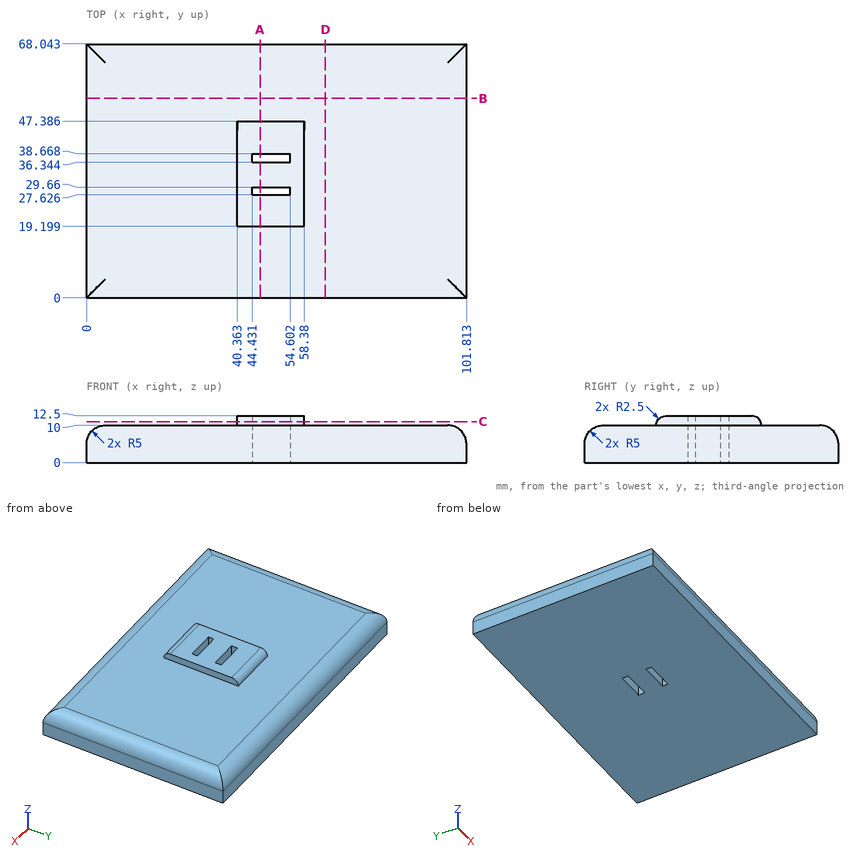
Geometry: see drawing. Coordinates: mm, zero at the bounding-box minimum. Coordinates: 2 decimals unless noted, no trailing zeros. Loops run counter-clockwise (first coordinate to the right, second up) from the corner with the lowest first, then second, coordinate; pieces in that order, holes last. Notation, with made-up numbers: (-11.75, -6) - (43.25, -6) arc R20 cw to (43.25, 1) - close; hole circle Ø4 at (-14.75, 73). An arc over 180 degrees is marked (long way). Put each result on its own line as item: value. Start each with the question number.
Q1. Cut plane C-C, the plane z = 11. Return loops of the section in (x, y).
Q2. Line query: line 1 (Y direction, x = 51.5, z = 2.5); line 2 (X direction, y = 28.5, z = 1); line 3 (X direction, y = 22, z = 11). Output: solid intervals per line, ascending.
Q3. Cut plane A-A, the plane x = 46.5. Give the number of separate pieces and of enclosed holes in the cut face, and give its area (3 significant figures).
Q4. Cut plane D-D, the plane x = 64. Return loops of the section in (y, z).
Q5. Cut plane B-B, the plane y = 53.5. Return loops of the section in (x, z), and give its area (3 significant figures).
Q6. Pin query (flat end, axial travel): pin 1 Ø3 at (x, z) = (31.5, 8) entering from +Y; pin 2 Ø5 at (x, y) = (27.5, 24) entering from +Z; pin 3 Ø1.2 at (y, z) = (38, 9) entering from +X. Return the tip coordinate at first contact, or that it passes through.
Filled sheet:
1. outline: (40.36, 19.41) - (58.38, 19.41) - (58.38, 47.18) - (40.36, 47.18) - close; hole (44.43, 27.63) - (54.6, 27.63) - (54.6, 29.66) - (44.43, 29.66) - close; hole (44.43, 36.34) - (54.6, 36.34) - (54.6, 38.67) - (44.43, 38.67) - close
2. line 1: 0 to 27.63, 29.66 to 36.34, 38.67 to 68.04
2. line 2: 0 to 44.43, 54.6 to 101.81
2. line 3: 40.36 to 58.38
3. separate pieces: 3
3. enclosed holes: 0
3. area: 683 mm²
4. outline: (0, 0) - (68.04, 0) - (68.04, 5) arc R5 ccw to (63.04, 10) - (5, 10) arc R5 ccw to (0, 5) - close
5. outline: (0, 0) - (101.81, 0) - (101.81, 5) arc R5 ccw to (96.81, 10) - (5, 10) arc R5 ccw to (0, 5) - close
5. area: 1,010 mm²
6. pin 1: y = 67.81
6. pin 2: z = 10
6. pin 3: x = 100.48
